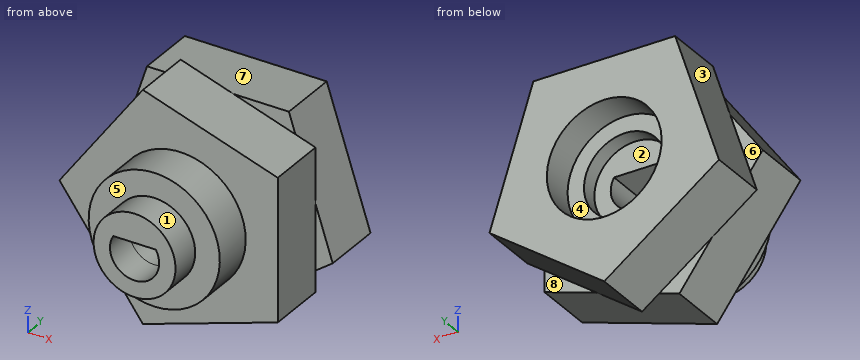
```python
from build123d import *
from build123d.topology import SkipClean

# Parameters (mm, degrees)
EXTRUDE_1_DEPTH     = 3.65
EXTRUDE_2_DEPTH     = 3.65
SKETCH_3_R          = 3.5
CUT_EXTRUDE_1_DEPTH = 2
SKETCH_4_R          = 4
EXTRUDE_3_DEPTH     = 2.5
CUT_EXTRUDE_2_DEPTH = 15.296125349
SKETCH_7_R          = 2.5
CUT_EXTRUDE_3_DEPTH = 1
SKETCH_8_R          = 2.5
EXTRUDE_4_DEPTH     = 1.9


with BuildPart() as part:
    # 草图1 → 凸台-拉伸1 (new body)
    with BuildSketch(Plane(origin=(0, 0, 0), x_dir=(1, 0, 0), z_dir=(0, 1, 0))):
        Polygon((0, 7.36), (-6.99977596, 2.274365079), (-4.326099457, -5.954365079), (4.326099457, -5.954365079), (6.99977596, 2.274365079), align=None)
    extrude(amount=EXTRUDE_1_DEPTH)

    # 草图2 → 凸台-拉伸2 (add)
    with BuildSketch(Plane(origin=(0, 0, 0), x_dir=(1, 0, 0), z_dir=(0, 1, 0))):
        Polygon((-2.274365079, -6.99977596), (5.954365079, -4.326099457), (5.954365079, 4.326099457), (-2.274365079, 6.99977596), (-7.36, 0), align=None)
    extrude(amount=-EXTRUDE_2_DEPTH)

    # 草图3 → 切除-拉伸1 (cut)
    with BuildSketch(Plane(origin=(0, 3.65, 0), x_dir=(1, 0, 0), z_dir=(0, 1, 0))):
        with Locations(Location((0, 0, 0), (0, 0, 270))):
            Circle(SKETCH_3_R)
    extrude(amount=-CUT_EXTRUDE_1_DEPTH, mode=Mode.SUBTRACT)

    # 草图4 → 凸台-拉伸3 (add)
    with BuildSketch(Plane.XZ.offset(3.65)):
        with Locations(Location((0, 0, 0), (0, 0, 270))):
            Circle(SKETCH_4_R)
    extrude(amount=EXTRUDE_3_DEPTH)

    # 草图6 → 切除-拉伸2 (cut, through all)
    with BuildSketch(Plane.XZ.offset(6.15)):
        with BuildLine():
            Line((-1.299038106, 0.75), (1.299038106, 0.75))
            ThreePointArc((1.299038106, 0.75), (0, -1.5), (-1.299038106, 0.75))
        make_face()
    extrude(amount=-CUT_EXTRUDE_2_DEPTH, mode=Mode.SUBTRACT)

    # 草图7 → 切除-拉伸3 (cut)
    with BuildSketch(Plane(origin=(0, 1.65, 0), x_dir=(1, 0, 0), z_dir=(0, 1, 0))):
        with Locations(Location((0, 0, 0), (0, 0, 270))):
            Circle(SKETCH_7_R)
    extrude(amount=-CUT_EXTRUDE_3_DEPTH, mode=Mode.SUBTRACT)

    # 草图8 → 凸台-拉伸4 (add)
    with SkipClean():  # the faces are left unmerged after this step: merging them gives an invalid solid
        with BuildSketch(Plane.XZ.offset(6.15)):
            with Locations(Location((0, 0, 0), (0, 0, 90))):
                Circle(SKETCH_8_R)
            with BuildLine():
                Line((1.299038106, 0.75), (-1.299038106, 0.75))
                ThreePointArc((-1.299038106, 0.75), (0, -1.5), (1.299038106, 0.75))
            make_face(mode=Mode.SUBTRACT)
        extrude(amount=EXTRUDE_4_DEPTH)


solid = part.part
```
Geometry: final body of the model. Coordinates: model frame, mm. Face numbers are marked on the shaded views. A direction names the side the tool comes from. Give positions to 0.01 mm unless a question says otherwise; leave off trailing zeros. Loops run counter-clockwise (first coordinate to the right, second up) from the corner with the lowest first, then second, coordinate; pieces in that order, holes last. Notation, with made-up numbers: (-6, 28) - (39, 28) arc R25 ccw to (39, 61) - close; hole circle Ø1 at (24, -15). An arc over 180 degrees is marked (long way). Answer as CSV lines item,"result". Start each with the question number.
(1) Section query D-D (z = 1.5). Output: boundary loops of the cut face in (x, y), and give its area (3 significant figures).
(2) Reachability of the marked faces 5, 6, 7 and 8 from +Z, -Z, +X, -X, +Y, -Y: full face, straight path, thin tool, end or side. Return the list, or none.
(3) Ray query, line 1 along X through (y, z) = (-6.75, 0); line 2 along Y through (x, z) = (3.75, 5.5); line 3 along Y through (x, z) = (5, -1.25). Return the intervals inside material, ascending. Write a range as [from, to].
(4) Section query C-C (y = 2.25). Output: boundary loops of the cut face in (x, z).
(5) Section query B-B (x = -0.75). Output: boundary loops of the cut face in (y, z).
(6) Mould query, pull axis X, two halves, no side actions, for the marked faces 1, 2, 3 and 4. Classes: +X half, -X half, draft (parallel to the pull), parting line (faces both ways), or undercut.
(7) Section query A-A (y = -2.75). Output: boundary loops of the cut face in (x, z).
(8) Pin query (flat end, axial travel): P1, Ø4, axis at x = 3.5, y = -3, coming from the +Z side; P2, Ø0.6, axis at x = 0, y = -7, coming from the -Z side; P3, Ø0.8, axis at x = 6.5, z = -1, coming from the -Y side; P4, Ø1.5, axis at y = -6, z = -5.5, coming from the +X side. Return the tip coordinate at first contact, or that it passes through.
Worked answers:
1,outline,"(-6.27, -3.65) - (-3.71, -3.65) - (-3.71, -6.15) - (-2, -6.15) - (-2, -8.05) - (2, -8.05) - (2, -6.15) - (3.71, -6.15) - (3.71, -3.65) - (5.95, -3.65) - (5.95, 0) - (5.77, 0) - (5.77, 3.65) - (3.16, 3.65) - (3.16, 1.65) - (2, 1.65) - (2, 0.65) - (-2, 0.65) - (-2, 1.65) - (-3.16, 1.65) - (-3.16, 3.65) - (-5.77, 3.65) - (-5.77, 0) - (-6.27, 0) - close"
1,area,"96.3 mm^2"
2,face 5,"-Y"
2,face 6,"+Z, -X, +Y"
2,face 7,"+Z, +X, -X, +Y"
2,face 8,"-Z, +X, +Y"
3,line 1,"x = [-2.5, -1.5], [1.5, 2.5]"
3,line 2,"y = [0, 3.65]"
3,line 3,"y = [-3.65, 3.65]"
4,outline,"(-7, -2.27) - (0, -7.36) - (7, -2.27) - (4.33, 5.95) - (-4.33, 5.95) - close; hole circle Ø7 at (0, 0)"
5,outline,"(-8.05, -2.38) - (-6.15, -2.38) - (-6.15, -3.93) - (-3.65, -3.93) - (-3.65, -6.5) - (0, -6.5) - (0, -6.82) - (3.65, -6.82) - (3.65, -3.42) - (1.65, -3.42) - (1.65, -2.38) - (0.65, -2.38) - (0.65, -1.3) - (-8.05, -1.3) - close; (-8.05, 0.75) - (0.65, 0.75) - (0.65, 2.38) - (1.65, 2.38) - (1.65, 3.42) - (3.65, 3.42) - (3.65, 5.95) - (0, 5.95) - (0, 6.5) - (-3.65, 6.5) - (-3.65, 3.93) - (-6.15, 3.93) - (-6.15, 2.38) - (-8.05, 2.38) - close"
6,face 1,"parting line"
6,face 2,"undercut"
6,face 3,"-X half"
6,face 4,"undercut"
7,outline,"(-7.36, 0) - (-2.27, -7) - (5.95, -4.33) - (5.95, 4.33) - (-2.27, 7) - close; hole (-1.3, 0.75) arc R1.5 ccw (long way) to (1.3, 0.75) - close"
8,P1,"stops at z = 5.77"
8,P2,"stops at z = -2.5"
8,P3,"stops at y = 0"
8,P4,"passes through"
